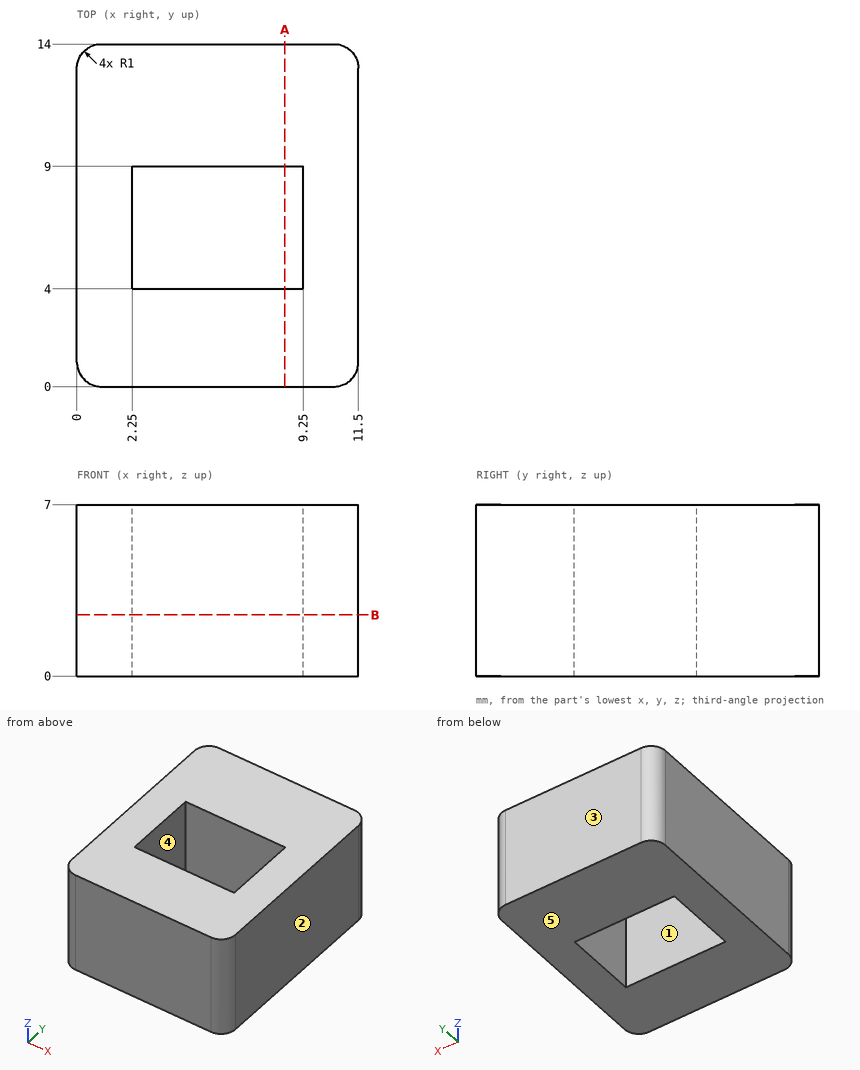
Verification items for this drawing (mm, ordinates from the low corner). A direction names the side the tool comes from. Coordinates: 2 decimals unless noted, no trailing zeros. Order: outer loops, then holes, each group sorted by start corner. A loop starts at its lowest first (then second) coordinate and runs counter-clockwise, first axis right, second up.
Q1. Sectioned sample at A-A on x = 8.5. Record the cut outline in (y, z).
Reply:
outline: (0, 0) - (4, 0) - (4, 7) - (0, 7) - close; (9, 0) - (14, 0) - (14, 7) - (9, 7) - close
Q2. Thickness scan on probe 1 along Y at (x, z) = (3.25, 1.5); probe 2 along X at (y, z) = (7.25, 2); probe 3 along X at (y, z) = (13.25, 3). Record the ranges inside material, lowest first.
Reply:
probe 1: y = 0 to 4, 9 to 14
probe 2: x = 0 to 2.25, 9.25 to 11.5
probe 3: x = 0.03 to 11.47
Q3. Tool access check on the marked faces 1 and 2. Record the directions out of +Z, -Z, +X, -X, +Y, -Y that give a thin tool (end or side, any length) a straight path to the whole face; none if there is none.
Reply:
face 1: +Z, -Z
face 2: +Z, -Z, +X, +Y, -Y
Q4. Sectioned sample at B-B on z = 2.5. Record the cut outline in (x, y), and give its area (3 significant figures).
Reply:
outline: (0, 1) arc R1 ccw to (1, 0) - (10.5, 0) arc R1 ccw to (11.5, 1) - (11.5, 13) arc R1 ccw to (10.5, 14) - (1, 14) arc R1 ccw to (0, 13) - close; hole (2.25, 4) - (9.25, 4) - (9.25, 9) - (2.25, 9) - close
area: 125 mm2
Q5. Draft check along Y on the marked faces 3, 4 and 5. Enter one of: released by +Y, released by -Y, zero draft, split by the parting line, or undercut.
Reply:
face 3: released by +Y
face 4: undercut
face 5: zero draft
